```python
from build123d import *

# Parameters (mm, degrees)
F0_W     = 150
F0_H     = 150
F0_R     = 3
F1_DEPTH = 1.5
F2_DEPTH = 20


with BuildPart() as f1:
    # F0 (on Top) → F1 (new body)
    with BuildSketch(Plane.XY):
        with Locations((-8.750431, 30.283519)):
            Rectangle(F0_W, F0_H)
        with Locations((-41.250431, 70.283519)):
            Circle(F0_R, mode=Mode.SUBTRACT)
        with Locations((23.749569, 70.283519)):
            Circle(F0_R, mode=Mode.SUBTRACT)
    extrude(amount=F1_DEPTH)

    # F0 (on Top) → F2 (join)
    with BuildSketch(Plane.XY):
        with Locations((-41.250431, 70.283519)):
            Circle(F0_R)
        with Locations((23.749569, 70.283519)):
            Circle(F0_R)
    extrude(amount=F2_DEPTH)


solid = f1.part
```
Input: part model. Units: mm. Frame: model coordinates. A direction names the side the tool comes from. Round coordinates to 2 decimals unless told otherwise and drop trailing zeros. Write each loop counter-clockwise with the first axis right and the second up, starting at its lowest first coordinate (ties: lowest second). Pieces come first, ordered by that corner, then holes. Notation, with made-up numbers: (-30.75, 40) -> (-21.75, 40) arc R18 cw to (-21.75, 47) -> close; hole circle Ø9 at (20, -24.5). An arc over 180 degrees is marked (long way). Answer as CSV lines item,"result".
1. Section A-A (x = -65.5). Return the cut outline in (y, z).
Geometry says:
outline,"(-44.72, 0) -> (105.28, 0) -> (105.28, 1.5) -> (-44.72, 1.5) -> close"
2. Contact query for flat-ended pins moving along their axis: P1, Ø8, axis at x = -44.5, z = 16.5, coming from the -Y side; P2, Ø4, axis at x = -55.5, y = 65.5, coming from the +Z side. Output: stop coordinate, or through.
Geometry says:
P1,"stops at y = 67.28"
P2,"stops at z = 1.5"
3. Section B-B (z = 12.5). Return the cut outline in (x, y).
Geometry says:
outline,"circle Ø6 at (-41.25, 70.28); circle Ø6 at (23.75, 70.28)"
4. Ray query, L1, parallel to Z at x = 26.5, y = 20; L2, parallel to Y at x = -40, z = 15.5; L3, parallel to Y at x = 26, z = 5. Return the intervals inside material, ascending. Write a range as [from, to].
Geometry says:
L1,"z = [0, 1.5]"
L2,"y = [67.56, 73.01]"
L3,"y = [68.3, 72.27]"
5. Reachability of faces 1 (the flat face through (-10, 31, 0)), 2 (the cylindrical face through (-43.46, 72.31, 10.62)) from +Z, -Z, +X, -X, +Y, -Y: full face, straight path, thin tool, end or side. Return the list, or none.
Geometry says:
face 1,"-Z, +X, -X, +Y, -Y"
face 2,"+Z"
6. Section C-C (y = 78.5). Return the cut outline in (x, z).
Geometry says:
outline,"(-83.75, 0) -> (66.25, 0) -> (66.25, 1.5) -> (-83.75, 1.5) -> close"
